from build123d import *

# Parameters (mm, degrees)
F0_W     = 50.8
F0_H     = 50.8
F0_W_2   = 19.05
F0_H_2   = 19.05
F1_DEPTH = 3.175


with BuildPart() as f1:
    # F0 (on Front) → F1 (new body)
    with BuildSketch(Plane.XZ):
        Polygon((185.420972, 200.016092), (-170.179028, 200.016092), (-170.179028, -130.183908), (-132.079028, -130.183908), (-81.279028, -130.197912), (-81.279028, -15.883908), (-132.079028, -15.883908), (-132.079028, 47.616092), (-5.079028, 47.616092), (-5.079028, -130.183908), (7.620972, -130.183908), (7.620972, -53.983908), (58.420972, -53.983908), (58.420972, -130.183908), (185.420972, -130.183908), (185.420972, 114.291092), align=None)
        with Locations((147.320972, 73.016092)):
            Rectangle(F0_W, F0_H, mode=Mode.SUBTRACT)
        with Locations((58.420972, 123.816092)):
            Rectangle(F0_W_2, F0_H_2, mode=Mode.SUBTRACT)
    extrude(amount=F1_DEPTH)


solid = f1.part
The listing builds one solid part. Answer for the finished solid, in the listing's coordinates (mm). Coordinates: 2 decimals unless noted, no trailing zeros. Write each loop counter-clockwise with the first axis right and the second up, starting at its lowest first coordinate (ties: lowest second). Pieces come first, ordered by that corner, then holes. Notation, with made-up numbers: M 13.25,-23.5 L 24.25,-23.5 A21 cw 24.25,11.5 Z; hole C 1.5,84 d6. An arc over 180 degrees is marked long. Put each result on its own line as item: value. Start each with the question number.
1. A flat-ended cylindrical pin translates along its axis: P1, Ø1, axis at x = 3, y = -2, coming from the -Z side. Find the tip coordinate at first contact, or state that the pin passes through.
2. A cutting plane is placed at A-A on y = -2.05. Write down the section's boundary in (x, z).
3. A cutting plane is placed at C-C on x = 53.5. Write down the section's boundary in (y, z) (3 decimals).
4. Consider line 1 (X direction, y = -3, z = -62); line 2 (Z direction, x = 160.5, y = -0.5); line 3 (Z direction, x = 65, y = -0.55). Determine where each line is inside the solid, lowest interval first. Write a range as from..to.
5. A cutting plane is placed at D-D on x = -61. Write down the section's boundary in (y, z) (3 decimals).
6. A cutting plane is placed at B-B on z = -40.5. Write down the section's boundary in (x, y) (3 decimals).
Resolved:
1. P1: stops at z = -130.18
2. outline: M -170.18,-130.18 L -132.08,-130.18 L -81.28,-130.2 L -81.28,-15.88 L -132.08,-15.88 L -132.08,47.62 L -5.08,47.62 L -5.08,-130.18 L 7.62,-130.18 L 7.62,-53.98 L 58.42,-53.98 L 58.42,-130.18 L 185.42,-130.18 L 185.42,200.02 L -170.18,200.02 Z; hole M 48.9,114.29 L 67.95,114.29 L 67.95,133.34 L 48.9,133.34 Z; hole M 121.92,47.62 L 172.72,47.62 L 172.72,98.42 L 121.92,98.42 Z
3. outline: M -3.175,-53.984 L 0,-53.984 L 0,114.291 L -3.175,114.291 Z; M -3.175,133.341 L 0,133.341 L 0,200.016 L -3.175,200.016 Z
4. line 1: x = -170.18..-81.28, -5.08..7.62, 58.42..185.42
4. line 2: z = -130.18..47.62, 98.42..200.02
4. line 3: z = -130.18..114.29, 133.34..200.02
5. outline: M -3.175,47.616 L 0,47.616 L 0,200.016 L -3.175,200.016 Z
6. outline: M -170.179,-3.175 L -81.279,-3.175 L -81.279,0 L -170.179,0 Z; M -5.079,-3.175 L 185.421,-3.175 L 185.421,0 L -5.079,0 Z
